The drawing under review shows one solid part. Ordinate dimensions are in mm from its lowest x, y, z. Coordinates: 2 decimals unless noted, no trailing zeros. Write each loop counter-clockwise with the first axis right and the second up, starting at its lowest first coordinate (ties: lowest second). Pieces come first, ordered by that corner, then holes.
Q1. Add section C-C, the plane y = 129.54. Give the boundary of the cut face in (x, z), plus the area to 3 significant figures.
Q2. Add section B-B, the plane x = 95. Give the boundary of the cut face in (y, z), plus the area to 3 significant figures.
Q3. To check wall thickness, follow probe 1 along Y at (x, z) = (100.33, 1); probe 2 along Y at (x, z) = (2.5, 6.35); probe 3 along Y at (x, z) = (81, 1.75). State the ranges of each line that lie inside material, in increasing order.
Q4. Clearance check with flat-ended pins moving along their axes: pin 1 Ø3 at (x, y) = (38, 130) entering from +Z; pin 2 Ø1.1 at (x, z) = (3.5, 5.5) entering from -Y. State where each tip first meets the part, or that it passes through.
Q5. Add section A-A, the plane y = 53.34. Give the boundary of the cut face in (x, z).
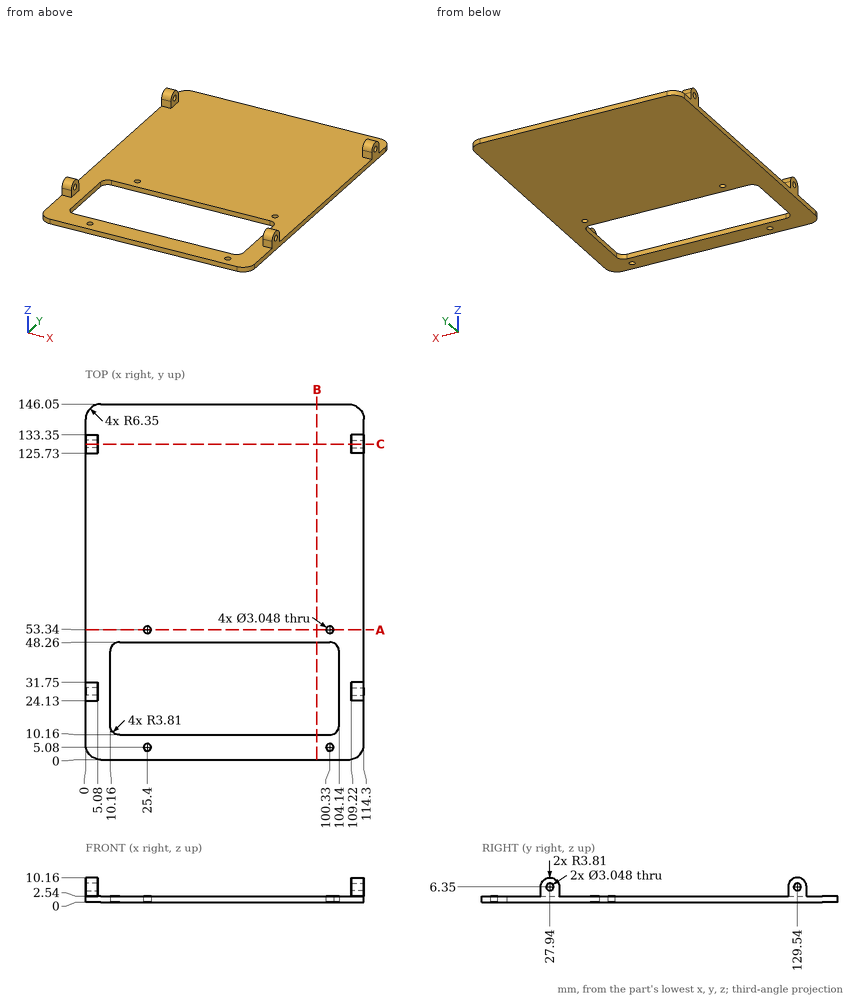
Here are the results:
1. outline: (0, 0) - (114.3, 0) - (114.3, 4.83) - (109.22, 4.83) - (109.22, 2.54) - (5.08, 2.54) - (5.08, 4.83) - (0, 4.83) - close; (0, 7.87) - (5.08, 7.87) - (5.08, 10.16) - (0, 10.16) - close; (109.22, 7.87) - (114.3, 7.87) - (114.3, 10.16) - (109.22, 10.16) - close
1. area: 337 mm2
2. outline: (0, 0) - (10.16, 0) - (10.16, 2.54) - (0, 2.54) - close; (48.26, 0) - (146.05, 0) - (146.05, 2.54) - (48.26, 2.54) - close
2. area: 274 mm2
3. probe 1: y = 0 to 3.56, 6.6 to 10.16, 48.26 to 51.82, 54.86 to 146.05
3. probe 2: y = 24.13 to 26.42, 29.46 to 31.75, 125.73 to 128.02, 131.06 to 133.35
3. probe 3: y = 0 to 10.16, 48.26 to 146.05
4. pin 1: stops at z = 2.54
4. pin 2: stops at y = 24.13
5. outline: (0, 0) - (23.88, 0) - (23.88, 2.54) - (0, 2.54) - close; (26.92, 0) - (98.81, 0) - (98.81, 2.54) - (26.92, 2.54) - close; (101.85, 0) - (114.3, 0) - (114.3, 2.54) - (101.85, 2.54) - close
